```python
from build123d import *

# Parameters (mm, degrees)
F0_R     = 1.1938
F1_DEPTH = 6.35
F2_R     = 5.08


with BuildPart() as f1:
    # F0 (on Top) → F1 (new body)
    with BuildSketch(Plane.XY):
        with BuildLine():
            ThreePointArc((38.1, 6.35), (0, 13.764279), (-38.1, 6.35))
            ThreePointArc((-38.1, 6.35), (-44.45, 0), (-38.1, -6.35))
            ThreePointArc((-38.1, -6.35), (0, 1.064279), (38.1, -6.35))
            ThreePointArc((38.1, -6.35), (44.45, 0), (38.1, 6.35))
        make_face()
        with Locations((-38.1, 0)):
            Circle(F0_R, mode=Mode.SUBTRACT)
        with Locations((38.1, 0)):
            Circle(F0_R, mode=Mode.SUBTRACT)
    extrude(amount=F1_DEPTH)

    # F2
    f2_edges = [f1.edges().sort_by_distance(p)[0] for p in [
        (-38.1, -6.35, 3.175),
        (38.1, -6.35, 3.175),
        (38.1, 6.35, 3.175),
        (-38.1, 6.35, 3.175),
    ]]
    fillet(f2_edges, radius=F2_R)


solid = f1.part
```
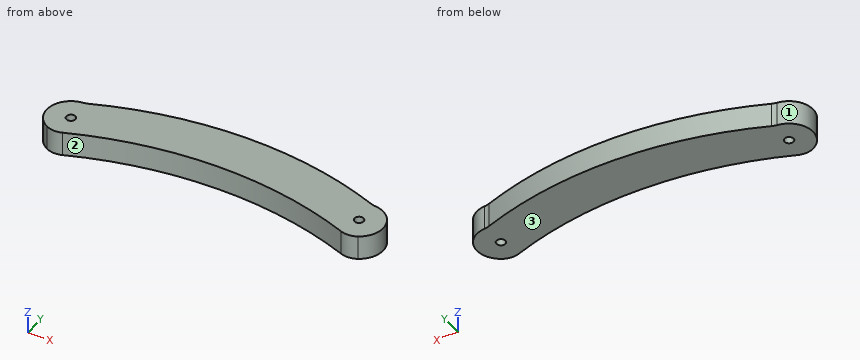
Here's how the part is built. I have some questions about the finished solid (model axes, mm). Face numbers are marked on the shaded views. Round coordinates to 2 decimals unless told otherwise and drop trailing zeros. Order: outer loops, then holes, each group sorted by start corner. A loop starts at its lowest first (then second) coordinate and runs counter-clockwise, first axis right, second up. Notation, with made-up numbers: M 66,-31.75 L 122,-31.75 A34 cw 122,-0.75 Z; hole C 84.25,28 d5. An arc over 180 degrees is marked long. Answer as CSV lines item,"result".
Item 1: Imagine slicing it at A-A on y = 0. List the corners of the cut face in (x, z) for me.
From the geometry:
outline,"M -44.45,0 L -39.29,0 L -39.29,6.35 L -44.45,6.35 Z; M -36.91,0 L -14.67,0 L -14.67,6.35 L -36.91,6.35 Z; M 14.67,0 L 36.91,0 L 36.91,6.35 L 14.67,6.35 Z; M 39.29,0 L 44.45,0 L 44.45,6.35 L 39.29,6.35 Z"
Item 2: Please list where these lines run through material, in increasing order: L1, parallel to Y at x = -38.1, z = 3.75; L2, parallel to X at y = 1.25, z = 0.5; L3, parallel to Y at x = 31, z = 4.75. Write a range as [from, to].
From the geometry:
L1,"[-6.17, -1.19], [1.19, 6.42]"
L2,"[-44.33, 44.33]"
L3,"[-3.78, 8.92]"
Item 3: For pin 1 (3 mm diameter, centred on y = -4, z = 4.5, fed in from +X); pin 2 (1 mm diameter, centred on y = 1.5, z = 5.5, fed in from -X), each with a flat end and sliding along its axis, tell me the tip position at first contact or that it passes through.
From the geometry:
pin 1,"x = 43.94"
pin 2,"x = -44.37"
Item 4: Imagine slicing it at B-B on y = -3.5. List the corners of the cut face in (x, z) for me, and give its area (3 significant figures).
From the geometry:
outline,"M -43.4,0 L -30.11,0 L -30.11,6.35 L -43.4,6.35 Z; M 30.11,0 L 43.4,0 L 43.4,6.35 L 30.11,6.35 Z"
area,"169 mm2"
Item 5: Imagine slicing it at C-C on z = 4. Give the number of separate pieces and of enclosed holes in the cut face, and give its area (3 significant figures).
From the geometry:
separate pieces,"1"
enclosed holes,"2"
area,"1,080 mm2"
Item 6: Imagine slicing it at D-D on x = 26.5. List the corners of the cut face in (y, z) for me.
From the geometry:
outline,"M -2.45,0 L 10.25,0 L 10.25,6.35 L -2.45,6.35 Z"
Item 7: We'd pull the mould along X, two halves only. Please class the marked faces 1, 2 and 3: +X half, -X half, draft (parallel to the pull), parting line (faces both ways), or undercut.
From the geometry:
face 1,"-X half"
face 2,"undercut"
face 3,"draft"
